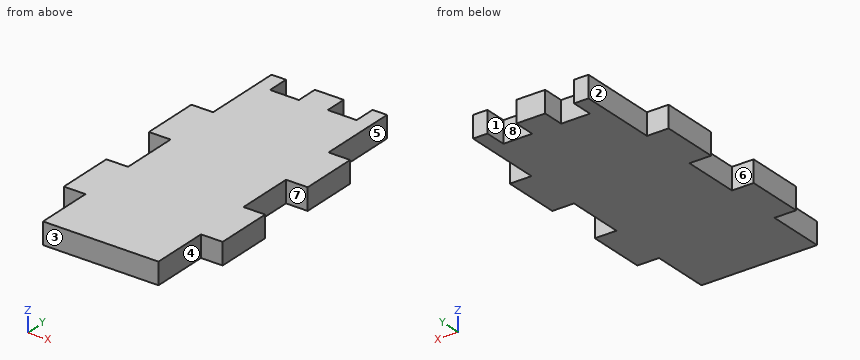
from build123d import *

# Parameters (mm, degrees)
F0_W     = 19.05
F0_H     = 50.8
F0_W_2   = 25.4
F0_H_2   = 19.05
F0_W_3   = 12.7
F1_DEPTH = 19.05


with BuildPart() as f1:
    # F0 (on Top) → F1 (new body)
    with BuildSketch(Plane.XY):
        with Locations((-111.125, 60.1353453214)):
            Rectangle(F0_W, F0_H)
        with Locations((-111.125, -41.4646546786)):
            Rectangle(F0_W, F0_H)
        Polygon((-88.9, 136.3353453214), (-101.6, 136.3353453214), (-101.6, 85.5353453214), (-101.6, 34.7353453214), (-101.6, -16.0646546786), (-101.6, -66.8646546786), (-101.6, -117.6646546786), (0, -117.6646546786), (0, -101.2241342793), (0, -66.8646546786), (0, -16.0646546786), (0, 34.7353453214), (0, 85.5353453214), (0, 136.3353453214), (-12.7, 136.3353453214), (-25.4, 136.3353453214), (-38.1, 136.3353453214), (-63.5, 136.3353453214), align=None)
        with Locations((9.525, -41.4646546786)):
            Rectangle(F0_W, F0_H)
        with Locations((9.525, 60.1353453214)):
            Rectangle(F0_W, F0_H)
        with Locations((-50.8, 145.8603453214)):
            Rectangle(F0_W_2, F0_H_2)
        with Locations((-95.25, 145.8603453214)):
            Rectangle(F0_W_3, F0_H_2)
        with Locations((-6.35, 145.8603453214)):
            Rectangle(F0_W_3, F0_H_2)
    extrude(amount=F1_DEPTH)


solid = f1.part
Design review of the part built by this model. Coordinates are the model's own, in mm. Face numbers are marked on the shaded views. A direction names the side the tool comes from. Give positions to 0.01 mm unless a question says otherwise; leave off trailing zeros. Order: outer loops, then holes, each group sorted by start corner. A loop starts at its lowest first (then second) coordinate and runs counter-clockwise, first axis right, second up. Notation, with made-up numbers: (34, 68) - (76, 68) arc R15 cw to (76, 87) - close; hole circle Ø3 at (29.5, 26.25). An arc over 180 degrees is marked (long way). Use CSV: the item, a comma, the result in double quotes. Start each with the question number.
Q1. Take a section at D-D (x = -30.5). State the section outline as (y, z) points.
Q2. Take a section at A-A (x = 4). State the section outline as (y, z) points.
Q3. Draft analysis for pull direction X (two halves, no side actions). For the marked faces 1, 2 and 3, state which applies: pulls with the +X half, pulls with the -X half, needs draft (parallel to the pull), parting line crosses it, or undercut.
Q4. Take a section at C-C (y = 92). State the section outline as (x, z) points.
Q5. For line 1 (Y direction, x = -112, z = 12.25); line 2 (X direction, y = 92, z = 4.5); line 3 (Y direction, x = -64, z = 2.25), list the stretches that pass through material, from the lowest coordinate up.
Q6. Machinability: for the marked faces 4, 5, 6, 7 and 8, which of the approach directions +Z, -Z, +X, -X, +Y, -Y give a long, thin tool a straight path to every point of the face, cutting with its end or side? Answer none if there is none.
Q7. For P1, Ø9.5, axis at y = 6, z = 11.5, coming from the -X side; P2, Ø5.5, axis at x = 8, z = 9.5, coming from the +Y side; P3, Ø4, axis at y = 10, z = 7.5, coming from the +X side, all flat-tipped, find the tip position at first contact; note any pin that passes through.
Q8. Take a section at B-B (z = 6.25). State the section outline as (x, y) points, and give its area (3 significant figures).
Calculated:
1,outline,"(-117.66, 0) - (136.34, 0) - (136.34, 19.05) - (-117.66, 19.05) - close"
2,outline,"(-66.86, 0) - (-16.06, 0) - (-16.06, 19.05) - (-66.86, 19.05) - close; (34.74, 0) - (85.54, 0) - (85.54, 19.05) - (34.74, 19.05) - close"
3,face 1,"undercut"
3,face 2,"pulls with the -X half"
3,face 3,"needs draft"
4,outline,"(-101.6, 0) - (0, 0) - (0, 19.05) - (-101.6, 19.05) - close"
5,line 1,"y = -66.86 to -16.06, 34.74 to 85.54"
5,line 2,"x = -101.6 to 0"
5,line 3,"y = -117.66 to 136.34"
6,face 4,"+Z, -Z, +X, -Y"
6,face 5,"+Z, -Z, +X, +Y"
6,face 6,"+Z, -Z, -X"
6,face 7,"+Z, -Z, +X"
6,face 8,"+Z, -Z, +Y"
7,P1,"stops at x = -101.6"
7,P2,"stops at y = 85.54"
7,P3,"stops at x = 0"
8,outline,"(-120.65, -66.86) - (-101.6, -66.86) - (-101.6, -117.66) - (0, -117.66) - (0, -66.86) - (19.05, -66.86) - (19.05, -16.06) - (0, -16.06) - (0, 34.74) - (19.05, 34.74) - (19.05, 85.54) - (0, 85.54) - (0, 155.39) - (-12.7, 155.39) - (-12.7, 136.34) - (-38.1, 136.34) - (-38.1, 155.39) - (-63.5, 155.39) - (-63.5, 136.34) - (-88.9, 136.34) - (-88.9, 155.39) - (-101.6, 155.39) - (-101.6, 85.54) - (-120.65, 85.54) - (-120.65, 34.74) - (-101.6, 34.74) - (-101.6, -16.06) - (-120.65, -16.06) - close"
8,area,"30,600 mm²"
